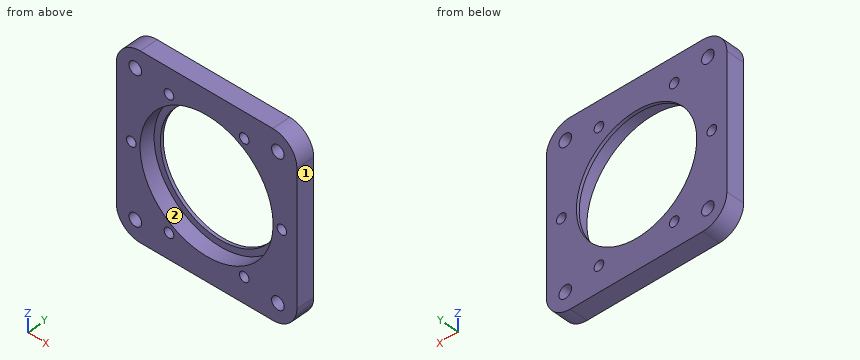
```python
from build123d import *

# Parameters (mm, degrees)
SKETCH_1_W          = 60
SKETCH_1_H          = 60
SKETCH_1_R          = 20
EXTRUDE_1_DEPTH     = 6
SKETCH_3_R          = 22.1
CUT_EXTRUDE_1_DEPTH = 5
SKETCH_4_R          = 1.6
SKETCH_4_R_2        = 2.1
CUT_EXTRUDE_2_DEPTH = 6
FILLET_1_R          = 8


with BuildPart() as part:
    # 草图1 → 凸台-拉伸1 (new body)
    with BuildSketch(Plane(origin=(0, 0, 0), x_dir=(1, 0, 0), z_dir=(0, 1, 0))):
        Rectangle(SKETCH_1_W, SKETCH_1_H)
        with Locations(Location((0, 0, 0), (0, 0, 270))):
            Circle(SKETCH_1_R, mode=Mode.SUBTRACT)
    extrude(amount=EXTRUDE_1_DEPTH)

    # 草图3 → 切除-拉伸1 (cut)
    with BuildSketch(Plane.XZ):
        with Locations(Location((0, 0, 0), (0, 0, 270))):
            Circle(SKETCH_3_R)
    extrude(amount=-CUT_EXTRUDE_1_DEPTH, mode=Mode.SUBTRACT)

    # 草图4 → 切除-拉伸2 (cut)
    with BuildSketch(Plane(origin=(0, 6, 0), x_dir=(1, 0, 0), z_dir=(0, 1, 0))):
        with Locations(Location((25, 0, 0), (0, 0, 270))):
            Circle(SKETCH_4_R)
        with Locations(Location((12.5, -21.650635095, 0), (0, 0, 270))):
            Circle(SKETCH_4_R)
        with Locations(Location((-12.5, -21.650635095, 0), (0, 0, 270))):
            Circle(SKETCH_4_R)
        with Locations(Location((-25, 0, 0), (0, 0, 270))):
            Circle(SKETCH_4_R)
        with Locations(Location((-12.5, 21.650635095, 0), (0, 0, 270))):
            Circle(SKETCH_4_R)
        with Locations(Location((12.5, 21.650635095, 0), (0, 0, 270))):
            Circle(SKETCH_4_R)
        with Locations(Location((23.68807717, 23.68807717, 0), (0, 0, 270))):
            Circle(SKETCH_4_R_2)
        with Locations(Location((23.68807717, -23.68807717, 0), (0, 0, 270))):
            Circle(SKETCH_4_R_2)
        with Locations(Location((-23.68807717, -23.68807717, 0), (0, 0, 270))):
            Circle(SKETCH_4_R_2)
        with Locations(Location((-23.68807717, 23.68807717, 0), (0, 0, 270))):
            Circle(SKETCH_4_R_2)
    extrude(amount=-CUT_EXTRUDE_2_DEPTH, mode=Mode.SUBTRACT)

    # 圆角1
    fillet_1_edges = [part.edges().sort_by_distance(p)[0] for p in [
        (30, 3, 30),
        (-30, 3, 30),
        (-30, 3, -30),
        (30, 3, -30),
    ]]
    fillet(fillet_1_edges, radius=FILLET_1_R)


solid = part.part
```
The model under review builds one solid part; all positions refer to its coordinate system, in mm. Face numbers are marked on the shaded views. A direction names the side the tool comes from. Give positions to 0.01 mm unless a question says otherwise; leave off trailing zeros. Write each loop counter-clockwise with the first axis right and the second up, starting at its lowest first coordinate (ties: lowest second). Pieces come first, ordered by that corner, then holes. Notation, with made-up numbers: (-32.5, 6.5) - (20.5, 6.5) arc R9 cw to (20.5, 15.5) - close; hole circle Ø3 at (28.25, 6.25). An arc over 180 degrees is marked (long way). Answer in a Markdown table with one row per item. Add a question column.
1. Insertion check: P1, Ø22, axis at x = -1, z = 10, coming from the -Y side; P2, Ø5, axis at x = -12.5, z = -21.65, coming from the +Y side. Each pin has a flat end and moves straight along its axis. Give the tip position at first contact, or say it passes through.
2. We need section D-D on z = -9. Write out the cut boundary in (x, y), then the cut area to 3 significant figures.
3. We need section A-A on x = 0. Write out the cut boundary in (y, z), then the cut area to 3 significant figures.
4. Wall thickness on line 1 along X through (y, z) = (2.6, -24); line 2 along Z through (x, y) = (-17, 3.4); line 3 along X through (y, z) = (4.8, -12.5): over which ranges is each line inside the solid? List them lowest first. Write a range as [from, to].
5. We need section C-C on x = -12.5. Write out the cut boundary in (y, z).
6. Tool access review of the marked faces 1 and 2: name each direction out of +Z, -Z, +X, -X, +Y, -Y from which nothing blocks a thin tool from reaching the whole face with its end or side.
7. We need section B-B on z = 0. Write out the cut boundary in (x, y).
Ans:
| question | item | result |
|---|---|---|
| 1 | P1 | stops at y = 5 |
| 1 | P2 | stops at y = 6 |
| 2 | outline | (-30, 0) - (-20.18, 0) - (-20.18, 5) - (-17.86, 5) - (-17.86, 6) - (-30, 6) - close; (17.86, 5) - (20.18, 5) - (20.18, 0) - (30, 0) - (30, 6) - (17.86, 6) - close |
| 2 | area | 122 mm^2 |
| 3 | outline | (0, -30) - (6, -30) - (6, -20) - (5, -20) - (5, -22.1) - (0, -22.1) - close; (0, 22.1) - (5, 22.1) - (5, 20) - (6, 20) - (6, 30) - (0, 30) - close |
| 3 | area | 99.0 mm^2 |
| 4 | line 1 | x = [-29.75, -25.76], [-21.61, 21.61], [25.76, 29.75] |
| 4 | line 2 | z = [-30, -14.12], [14.12, 30] |
| 4 | line 3 | x = [-30, -18.23], [18.23, 30] |
| 5 | outline | (0, -30) - (6, -30) - (6, -23.25) - (0, -23.25) - close; (0, -20.05) - (6, -20.05) - (6, -15.61) - (5, -15.61) - (5, -18.23) - (0, -18.23) - close; (0, 18.23) - (5, 18.23) - (5, 15.61) - (6, 15.61) - (6, 20.05) - (0, 20.05) - close; (0, 23.25) - (6, 23.25) - (6, 30) - (0, 30) - close |
| 6 | face 1 | +Z, -Z, +X, +Y, -Y |
| 6 | face 2 | -Y |
| 7 | outline | (-30, 0) - (-26.6, 0) - (-26.6, 6) - (-30, 6) - close; (-23.4, 0) - (-22.1, 0) - (-22.1, 5) - (-20, 5) - (-20, 6) - (-23.4, 6) - close; (20, 5) - (22.1, 5) - (22.1, 0) - (23.4, 0) - (23.4, 6) - (20, 6) - close; (26.6, 0) - (30, 0) - (30, 6) - (26.6, 6) - close |
